```python
from build123d import *

# Parameters (mm, degrees)
SKETCH1_R               = 38
BOSS_EXTRUDE1_DEPTH     = 20
SKETCH2_R               = 28
SKETCH2_R_2             = 22.5
BOSS_EXTRUDE2_DEPTH     = 10
CUT_EXTRUDE1_DEPTH      = 58.341084747
CUT_EXTRUDE1_DEPTH_BACK = 58.341084747
SKETCH3_R               = 1.5


with BuildPart() as part:
    # Sketch1 → Boss-Extrude1 (new body)
    with BuildSketch(Plane(origin=(0, 0, 0), x_dir=(1, 0, 0), z_dir=(0, 1, 0))):
        with Locations(Location((0, 0, 0), (0, 0, 270))):
            Circle(SKETCH1_R)
    extrude(amount=BOSS_EXTRUDE1_DEPTH)

    # Sketch2 → Boss-Extrude2 (add)
    with BuildSketch(Plane.XZ):
        with Locations(Location((0, 0, 0), (0, 0, 90))):
            Circle(SKETCH2_R)
        with Locations(Location((0, 0, 0), (0, 0, 270))):
            Circle(SKETCH2_R_2, mode=Mode.SUBTRACT)
    extrude(amount=BOSS_EXTRUDE2_DEPTH)

    # Sketch3 → Cut-Extrude1 (cut, two sides: drawn at the far end of the back side and taken through both)
    with BuildSketch(Plane.XY.offset(-CUT_EXTRUDE1_DEPTH_BACK)):
        with Locations((32.986839826, 5)):
            Circle(SKETCH3_R)
        with Locations((32.986839826, 15)):
            Circle(SKETCH3_R)
        with Locations((-32.986839826, 5)):
            Circle(SKETCH3_R)
        with Locations((-32.986839826, 15)):
            Circle(SKETCH3_R)
    extrude(amount=CUT_EXTRUDE1_DEPTH + CUT_EXTRUDE1_DEPTH_BACK, mode=Mode.SUBTRACT)


solid = part.part
```
Build history of the part. All positions in model axes, mm. A direction names the side the tool comes from. Give positions to 0.01 mm unless a question says otherwise; leave off trailing zeros. Loops run counter-clockwise (first coordinate to the right, second up) from the corner with the lowest first, then second, coordinate; pieces in that order, holes last.
1) Band-saw the part on D-D on y = 5. List the corners of the cut face in (x, z), then the cut area to 3 significant figures.
Values follow:
outline: (-34.49, -15.96) - (-34.49, 15.96) arc R38 ccw to start; (-31.49, -21.27) arc R38 ccw to (31.49, -21.27) - (31.49, 21.27) arc R38 ccw to (-31.49, 21.27) - close; (34.49, -15.96) arc R38 ccw to (34.49, 15.96) - close
area: 4,310 mm2
2) 3-axis set-ups, long thin cutter, end or side, ignore diameter. For faces 1 (the face through (27.334, -4.93, -6.07)), 2 (the face through (-31.556, 5.451, -0.298)): which of +Z, -Z, +X, -X, +Y, -Y reach the whole face in a straight line?
Values follow:
face 1: -Y
face 2: +Z, -Z
3) Band-saw the part on C-C on y = -7.5. List the corners of the cut face in (x, z), then the cut area to 3 significant figures.
Values follow:
outline: circle Ø56 at (0, 0); hole circle Ø45 at (0, 0)
area: 873 mm2
4) Band-saw the part on B-B on x = 0. List the corners of the cut face in (y, z).
Values follow:
outline: (-10, -28) - (0, -28) - (0, -38) - (20, -38) - (20, 38) - (0, 38) - (0, 28) - (-10, 28) - (-10, 22.5) - (0, 22.5) - (0, -22.5) - (-10, -22.5) - close
5) Drop flat-ended pins along their axis: P1, Ø1.5, axis at y = 2, z = -7.5, coming from the -X side; P2, Ø10, axis at y = 13.5, z = 2, coming from the +X side; P3, Ø6, axis at x = -17.5, y = -4, coming from the +Z side. Give the stop position or say it passes through.
Values follow:
P1: stops at x = -37.4
P2: stops at x = 38
P3: stops at z = 23.95
6) Band-saw the part on A-A on z = 0. List the corners of the cut face in (x, y), then the cut area to 3 significant figures.
Values follow:
outline: (-38, 0) - (-28, 0) - (-28, -10) - (-22.5, -10) - (-22.5, 0) - (22.5, 0) - (22.5, -10) - (28, -10) - (28, 0) - (38, 0) - (38, 20) - (-38, 20) - close; hole circle Ø3 at (-32.99, 5); hole circle Ø3 at (-32.99, 15); hole circle Ø3 at (32.99, 5); hole circle Ø3 at (32.99, 15)
area: 1,600 mm2
7) Probe line 1 along X through (y, z) = (15, 8.5); line 2 along X through (y, z) = (6, 0.5); line 3 along Y through (x, z) = (-4.5, -5). List the from-to ranges inside material, lowest first.
Values follow:
line 1: x = -37.04 to -34.49, -31.49 to 31.49, 34.49 to 37.04
line 2: x = -38 to -34.1, -31.87 to 31.87, 34.1 to 38
line 3: y = 0 to 20
8) Two-plate mould, pull along Z, no slides. Class faces 3 (the face through (31.49, 5.07, -0.3)), 4 (the face through (1.671, 9.86, -37.963)), 5 (the face through (-8.618, -4.93, -20.784)): released by +Z, released by -Z, zero draft, split by the parting line, or undercut.
Values follow:
face 3: zero draft
face 4: split by the parting line
face 5: undercut
